```python
from build123d import *

# Parameters (mm, degrees)
F0_W     = 300
F0_H     = 500
F1_DEPTH = 18
F3_D     = 2.5
F3_DEPTH = 14.5
F3_TIP   = 0.7510757738
F5_D     = 2.5
F5_DEPTH = 14
F5_TIP   = 0.7510757738
F6_W     = 18
F6_H     = 1
F7_DEPTH = 500.001


with BuildPart() as f1:
    # F0 (on Top) → F1 (new body)
    with BuildSketch(Plane.XY):
        with Locations((150, -250)):
            Rectangle(F0_W, F0_H)
    extrude(amount=F1_DEPTH)

    # F3
    with Locations(Plane.XZ.offset(500)):
        with Locations((20, 9), (150, 9), (280, 9)):
            Hole(F3_D / 2, depth=F3_DEPTH)
            with Locations((0, 0, -(F3_DEPTH + F3_TIP / 2))):  # 118° drill point
                Cone(0, F3_D / 2, F3_TIP, mode=Mode.SUBTRACT)

    # F5
    with Locations(Plane(origin=(0, 0, 0), x_dir=(-1, 0, 0), z_dir=(0, 1, 0))):
        with Locations((-280, 9), (-150, 9), (-20, 9)):
            Hole(F5_D / 2, depth=F5_DEPTH)
            with Locations((0, 0, -(F5_DEPTH + F5_TIP / 2))):  # 118° drill point
                Cone(0, F5_D / 2, F5_TIP, mode=Mode.SUBTRACT)

    # F6 (on face) → F7 (cut, through all)
    with BuildSketch(Plane.XZ.offset(500)):
        with Locations((9, 17.5)):
            Rectangle(F6_W, F6_H)
        with Locations((9, 0.5)):
            Rectangle(F6_W, F6_H)
    extrude(amount=-F7_DEPTH, mode=Mode.SUBTRACT)


solid = f1.part
```
Input: part model. Units: mm. Frame: model coordinates. A direction names the side the tool comes from. Coordinates: 2 decimals unless noted, no trailing zeros.
Q1. Line query: line 1 along X through (y, z) = (-493.5, 9); line 2 along Z through (x, y) = (280, -4). Output: solid intervals per line, ascending.
Results are:
line 1: x = 0 to 18.75, 21.25 to 148.75, 151.25 to 278.75, 281.25 to 300
line 2: z = 0 to 7.75, 10.25 to 18
Q2. Contact query for flat-ended pins moving along their axis: pin 1 (3 mm diameter, centred on x = 280, z = 9, fed in from +Y); pin 2 (20 mm diameter, centred on x = 7.5, y = -130.5, fed in from -Z); pin 3 (2 mm diameter, centred on x = 20, z = 9, fed in from -Y); pin 4 (2 mm diameter, centred on x = 280, z = 9, fed in from +Y). Output: stop coordinate, or through.
Results are:
pin 1: stops at y = 0
pin 2: stops at z = 1
pin 3: stops at y = -485.35
pin 4: stops at y = -14.15
Q3. Set-up query: faces 1 (the flat face through (157, -246, 18)), 2 (the flat face through (9, -254, 1)), 3 (the flat face through (9, -254, 17)). Return all of +Z, -Z, +X, -X, +Y, -Y with unobstructed straight access to the full face (end or side cutting, diameter ignored); none if empty.
Results are:
face 1: +Z, +X, -X, +Y, -Y
face 2: -Z, -X, +Y, -Y
face 3: +Z, -X, +Y, -Y
